The model under review builds one solid part; all positions refer to its coordinate system, in mm. Round coordinates to 2 decimals unless told otherwise and drop trailing zeros. Write each loop counter-clockwise with the first axis right and the second up, starting at its lowest first coordinate (ties: lowest second). Pieces come first, ordered by that corner, then holes. Notation, with made-up numbers: (-1, 30) -> (8, 30) arc R23 cw to (8, 57) -> close; hole circle Ø5 at (59, 48). An arc over 180 degrees is marked (long way). Use CSV: the item, a comma, the result in double quotes. Start each with the question number.
1) Take a section at C-C, the plane x = 0. Give the boundary of the cut face in (y, z), then the cut area to 3 significant figures.
2) Take a section at B-B, the plane x = 180. Give the boundary of the cut face in (y, z).
3) For pin 1 Ø18 at (x, y) = (46.75, 0) entering from +Z; pin 2 Ø16 at (x, y) = (0, -46.75) entering from -Z, all flat-tipped, find the tip position at first contact; note any pin that passes through.
4) Take a section at D-D, the plane x = 46.75. Give the boundary of the cut face in (y, z).
5) Take a section at A-A, the plane z = -704.5. Give the boundary of the cut face in (x, y).
6) Wall thickness on probe 1 along Y at (x, z) = (0, 8.5); probe 2 along Y at (x, z) = (-46, 10); probe 3 along Z at (x, y) = (-27.5, 45.5): over which ranges is each line inside the solid? List them lowest first. Write a range as [from, to].
from build123d import *

# Parameters (mm, degrees)
F0_R     = 66.75
F1_DEPTH = 15
F2_R     = 20
F3_DEPTH = 1000
F5_DEPTH = 5
F6_R     = 10
F7_DEPTH = 50.8


with BuildPart() as f1:
    # F0 (on Top) → F1 (new body)
    with BuildSketch(Plane.XY):
        Circle(F0_R)
    extrude(amount=F1_DEPTH)

    # F2 (on face) → F3 (join)
    with BuildSketch(Plane(origin=(0, 0, 0), x_dir=(1, 0, 0), z_dir=(0, 0, -1))):
        Circle(F2_R)
    extrude(amount=F3_DEPTH)

    # F4 (on Front) → F5 (join, symmetric)
    with BuildSketch(Plane.XZ):
        Polygon((212.132034, -487.867966), (0, -700), (0, -740), (212.132034, -527.867966), align=None)
        Polygon((212.132034, -627.867966), (0, -840), (0, -880), (212.132034, -667.867966), align=None)
    extrude(amount=F5_DEPTH, both=True)

    # F6 (on face) → F7 (cut)
    with BuildSketch(Plane.XY.offset(15)):
        with Locations((0, -46.75)):
            Circle(F6_R)
        with Locations((46.75, 0)):
            Circle(F6_R)
        with Locations((0, 46.75)):
            Circle(F6_R)
        with Locations((-46.75, 0)):
            Circle(F6_R)
    extrude(amount=-F7_DEPTH, mode=Mode.SUBTRACT)


solid = f1.part
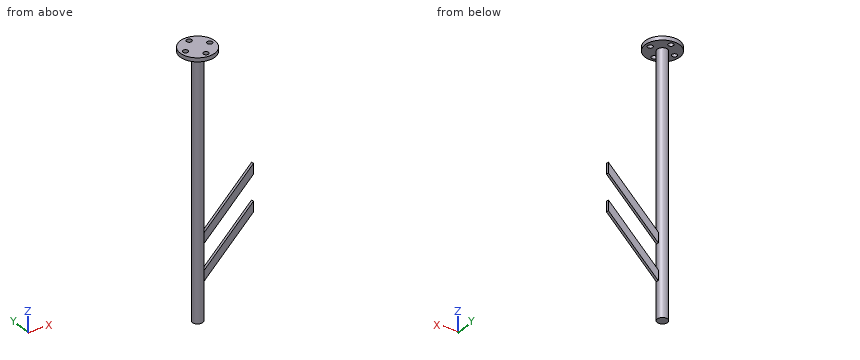
Values found:
1,outline,"(-66.75, 0) -> (-56.75, 0) -> (-56.75, 15) -> (-66.75, 15) -> close; (-36.75, 0) -> (-20, 0) -> (-20, -1000) -> (20, -1000) -> (20, 0) -> (36.75, 0) -> (36.75, 15) -> (-36.75, 15) -> close; (56.75, 0) -> (66.75, 0) -> (66.75, 15) -> (56.75, 15) -> close"
1,area,"41,400 mm²"
2,outline,"(-5, -700) -> (5, -700) -> (5, -660) -> (-5, -660) -> close; (-5, -560) -> (5, -560) -> (5, -520) -> (-5, -520) -> close"
3,pin 1,"z = -644.25"
3,pin 2,"through"
4,outline,"(-47.64, 0) -> (-10, 0) -> (-10, 15) -> (-47.64, 15) -> close; (-5, -833.25) -> (5, -833.25) -> (5, -793.25) -> (-5, -793.25) -> close; (-5, -693.25) -> (5, -693.25) -> (5, -653.25) -> (-5, -653.25) -> close; (10, 0) -> (47.64, 0) -> (47.64, 15) -> (10, 15) -> close"
5,outline,"(19.36, -5) -> (35.5, -5) -> (35.5, 5) -> (19.36, 5) arc R20 ccw (long way) to start; (135.5, -5) -> (175.5, -5) -> (175.5, 5) -> (135.5, 5) -> close"
6,probe 1,"[-66.75, -56.75], [-36.75, 36.75], [56.75, 66.75]"
6,probe 2,"[-48.37, -9.97], [9.97, 48.37]"
6,probe 3,"[0, 15]"
